Autodesk Inventor part; units mm, degrees
ref_plane "YZ Plane" through (0, 0, 0) normal (1, 0, 0) x (0, 1, 0)
ref_plane "XZ Plane" through (0, 0, 0) normal (0, 1, 0) x (-1, 0, 0)
ref_plane "XY Plane" through (0, 0, 0) normal (0, 0, 1) x (1, 0, 0)
sketch "Sketch1" plane through (0, 0, 0) normal (0, 1, 0) x (-1, 0, 0)
  circle A0 centre (0, 0) radius 4.318
  line L0 (0, -31.496) -> (5.08, -31.496)
  line L1 (0, -31.496) -> (-5.08, -31.496)
  line L2 (31.496, 0) -> (31.496, 5.08)
  line L3 (31.496, 0) -> (31.496, -5.08)
  line L4 (0, 31.496) -> (-5.08, 31.496)
  line L5 (0, 31.496) -> (5.08, 31.496)
  line L6 (-31.496, 0) -> (-31.496, -5.08)
  line L7 (-31.496, 0) -> (-31.496, 5.08)
  line L8 (31.496, 5.08) -> (50.5454, 5.08)
  line L9 (31.496, -5.08) -> (50.5454, -5.08)
  line L10 (5.08, -31.496) -> (5.08, -50.5454)
  line L11 (-5.08, -31.496) -> (-5.08, -50.5454)
  line L12 (-31.496, -5.08) -> (-50.5454, -5.08)
  line L13 (-31.496, 5.08) -> (-50.5454, 5.08)
  line L14 (-5.08, 31.496) -> (-5.08, 50.5454)
  line L15 (5.08, 31.496) -> (5.08, 50.5454)
  line L16 (-50.5454, 5.08) -> (-50.5454, 10.16)
  line L17 (-50.5454, -5.08) -> (-50.5454, -10.16)
  line L18 (-5.08, -50.5454) -> (-10.16, -50.5454)
  line L19 (5.08, -50.5454) -> (10.16, -50.5454)
  line L20 (50.5454, -5.08) -> (50.5454, -10.16)
  line L21 (50.5454, 5.08) -> (50.5454, 10.16)
  line L22 (5.08, 50.5454) -> (10.16, 50.5454)
  line L23 (-5.08, 50.5454) -> (-10.16, 50.5454)
  line L24 (-10.16, 50.5454) -> (-10.16, 29.8123)
  line L25 (10.16, 50.5454) -> (10.16, 29.8123)
  line L26 (-50.5454, 10.16) -> (-29.8123, 10.16)
  line L27 (-50.5454, -10.16) -> (-29.8123, -10.16)
  line L28 (-10.16, -50.5454) -> (-10.16, -29.8123)
  line L29 (10.16, -50.5454) -> (10.16, -29.8123)
  line L30 (50.5454, -10.16) -> (29.8123, -10.16)
  line L31 (50.5454, 10.16) -> (29.8123, 10.16)
  arc A1 (-10.16, 29.8123) -> (-29.8123, 10.16) centre (0, 0) ccw
  arc A2 (-29.8123, -10.16) -> (-10.16, -29.8123) centre (0, 0) ccw
  arc A3 (10.16, -29.8123) -> (29.8123, -10.16) centre (0, 0) ccw
  arc A4 (29.8123, 10.16) -> (10.16, 29.8123) centre (0, 0) ccw
  dimension "d7" = 360
  dimension "d13" = 360
  dimension "d0" = 8.636
  dimension "d9" = 5.08
  dimension "d10" = 5.08
extrude "Extrusion1" add sketch "Sketch1" along normal blind 7.62
sketch "Sketch2" plane through (10.16, 0, 50.5454) normal (1, 0, 0) x (0, 0, -1)
  line L0 (0, 0) -> (20.7331, 0)
  circle A0 centre (11.1754, 3.81) radius 1.651
  point P0 (50.5454, 0)
  dimension "d19" = 3.302
extrude "Extrusion2" cut sketch "Sketch2" against normal up to surface (20.32 mm away)
pattern_circular "Circular Pattern1" count 4 over 360 about axis through (0, 0, 0) along (0, 1, 0) of "Extrusion2"
sketch "Sketch3" plane through (0, 7.62, 0) normal (0, 1, 0) x (1, 0, 0)
  circle A0 centre (0, 0) radius 31.369
  circle A1 centre (0, 0) radius 11.2522
  dimension "d25" = 62.738
  dimension "d26" = 22.5044
extrude "Extrusion3" add sketch "Sketch3" along normal blind 4.826
sketch "Sketch4" plane through (0, 7.62, 0) normal (0, 1, 0) x (1, 0, 0)
  circle A0 centre (0, 0) radius 11.2522
extrude "Extrusion4" cut sketch "Sketch4" against normal blind 2.54
chamfer "Chamfer1" distance 3.175 angle 45 8 edges at (10.16, 3.81, 29.8123) (29.8123, 3.81, 10.16) (-10.16, 3.81, 29.8123) (-29.8123, 3.81, 10.16) (-29.8123, 3.81, -10.16) (-10.16, 3.81, -29.8123) (10.16, 3.81, -29.8123) (29.8123, 3.81, -10.16)
properties part number "center"
Here's how the part is built. I have some questions about the finished solid (model axes, mm). A direction names the side the tool comes from. Give positions to 0.01 mm unless a question says otherwise; leave off trailing zeros. Order: outer loops, then holes, each group sorted by start corner. A loop starts at its lowest first (then second) coordinate and runs counter-clockwise, first axis right, second up. Notation, with made-up numbers: (87.25, 89) -> (104.25, 89) arc R22 cw to (104.25, 126) -> close; hole circle Ø6 at (57, -37.5). An arc over 180 degrees is marked (long way). Use a Markdown table: item, result. Add a question column.
Item 1: For faces 4 (the face through (10.16, 4, -42)), 5 (the face through (41, 5, -5.08)), 6 (the face through (0, 5.08, 5)), which set-ups out of +Z, -Z, +X, -X, +Y, -Y let a thin tool reach every point of the face, with its end or its side?
Item 2: I need wall thicknesses on line 1 (Z direction, x = 36, y = 5); line 2 (Z direction, x = -6.5, y = 2.5); line 3 (Y direction, x = -7.3, z = 39.37). Which ranges of each line are inside material? Lowest first, please.
Item 3: If we mould it in two halves opening along Z, with no side actions, what happens to faces 1 (the face through (11.614, 3.757, -30.843)), 2 (the face through (8, 4, 50.545)), 3 (the face through (-41, 5, -5.08))? For each: pulls with the +Z half, pulls with the -Z half, needs draft (parallel to the pull), parting line crosses it, or undercut.
Item 4: Will these pins go through, and if not, where does the flat tip stop? pin 1 (6 mm diameter, centred on x = 30.5, y = 6.5, fed in from +Z); pin 2 (4 mm diameter, centred on y = 3.5, z = 39, fed in from -X); pin 3 (2.5 mm diameter, centred on x = -37, y = 4, fed in from -Z).
Item 5: Imagine slicing it at B-B on x = 39.37. Please give me the cut outline in (y, z).
Item 6: Imagine slicing it at D-D on z = 0. Please give me the cut outline in (x, y), plus the area to 3 significant figures.
Item 7: Imagine slicing it at A-A on z = 44. Please give me the cut outline in (x, y).
Item 8: Imagine slicing it at C-C on y = 3.81. Give the number of separate pieces and of enclosed holes in the cut face, plus the area to 3 significant figures.
Data:
| question | item | result |
|---|---|---|
| 1 | face 4 | -Z, +X, +Y, -Y |
| 1 | face 5 | +X, +Y, -Y |
| 1 | face 6 | +Y |
| 2 | line 1 | z = -10.16 to -5.08, 5.08 to 10.16 |
| 2 | line 2 | z = -50.55 to -40.37, -38.37 to 38.37, 40.37 to 50.55 |
| 2 | line 3 | y = 0 to 2.16, 5.46 to 7.62 |
| 3 | face 1 | pulls with the -Z half |
| 3 | face 2 | pulls with the +Z half |
| 3 | face 3 | undercut |
| 4 | pin 1 | stops at z = 15.35 |
| 4 | pin 2 | stops at x = -10.16 |
| 4 | pin 3 | stops at z = -10.16 |
| 5 | outline | (0, -10.16) -> (2.16, -10.16) -> (2.16, -5.08) -> (0, -5.08) -> close; (0, 5.08) -> (2.16, 5.08) -> (2.16, 10.16) -> (0, 10.16) -> close; (5.46, -10.16) -> (7.62, -10.16) -> (7.62, -5.08) -> (5.46, -5.08) -> close; (5.46, 5.08) -> (7.62, 5.08) -> (7.62, 10.16) -> (5.46, 10.16) -> close |
| 6 | outline | (-31.5, 0) -> (-4.32, 0) -> (-4.32, 5.08) -> (-11.25, 5.08) -> (-11.25, 12.45) -> (-31.37, 12.45) -> (-31.37, 7.62) -> (-31.5, 7.62) -> close; (4.32, 0) -> (31.5, 0) -> (31.5, 7.62) -> (31.37, 7.62) -> (31.37, 12.45) -> (11.25, 12.45) -> (11.25, 5.08) -> (4.32, 5.08) -> close |
| 6 | area | 573 mm² |
| 7 | outline | (-10.16, 0) -> (-5.08, 0) -> (-5.08, 7.62) -> (-10.16, 7.62) -> close; (5.08, 0) -> (10.16, 0) -> (10.16, 7.62) -> (5.08, 7.62) -> close |
| 8 | separate pieces | 9 |
| 8 | enclosed holes | 1 |
| 8 | area | 3,780 mm² |
